```python
from build123d import *

# Parameters (mm, degrees)
F0_W     = 50.8
F0_H     = 1219.2
F1_DEPTH = 25.4


with BuildPart() as f1:
    # F0 (on Right) → F1 (new body)
    with BuildSketch(Plane.YZ):
        Polygon((350.804755, -361.721163), (350.804755, -336.321163), (-182.595245, -336.321163), (-233.395245, -336.321163), (-487.395245, -336.321163), (-538.195245, -336.321163), (-538.195245, -361.721163), align=None)
        with Locations((-207.995245, 273.278837)):
            Rectangle(F0_W, F0_H)
        Polygon((-233.395245, 882.878837), (-182.595245, 882.878837), (-182.595245, 908.278837), (-538.195245, 908.278837), (-538.195245, 882.878837), (-487.395245, 882.878837), align=None)
        with Locations((-512.795245, 273.278837)):
            Rectangle(F0_W, F0_H)
    extrude(amount=F1_DEPTH)


solid = f1.part
```
Work out the finished part from the listing and answer in its coordinate system (mm). A direction names the side the tool comes from. Give positions to 0.01 mm unless a question says otherwise; leave off trailing zeros. Loops run counter-clockwise (first coordinate to the right, second up) from the corner with the lowest first, then second, coordinate; pieces in that order, holes last. Notation, with made-up numbers: (34, 45.25) -> (56, 45.25) arc R6 cw to (56, 53.25) -> close; hole circle Ø3 at (1, 80.25). An arc over 180 degrees is marked (long way). Put each result on its own line as item: value. Start each with the question number.
Item 1: Which of the six approach directions +Z, -Z, +X, -X, +Y, -Y give full straight-line access (tool end or side, diameter ignored) to faces 5 (the face through (13, -358, 908.279)), 6 (the face through (13, 88, -336.321)), 7 (the face through (13, -362, 882.879))?
Item 2: The part is cut by section B-B (x = 7.75). Give the vertices of the cut face in (y, z).
Item 3: The mould has two halves that part along Y. Classify faces 1 (the face through (13, -182.595, 277)), 2 (the face through (13, -233.395, 265)), 3 (the face through (13, -359, -336.321)), 4 (the face through (13, -100, -361.721)): released by +Y, released by -Y, zero draft, split by the parting line, or undercut.
Item 4: The part is cut by section A-A (z = 518). Give the vertices of the cut face in (x, y).
Item 5: Each of these flat-tipped pins is pushed along its axis until it touches: P1, Ø10, axis at x = 5.5, y = 79, coming from the +Z side; P2, Ø7.5, axis at x = 13, z = 123.5, coming from the +Y side. Where does it stop, or does it pass through?
Item 6: Find the intervals of material crossed by L1, parallel to Y at x = 21, z = 135; L2, parallel to Z at x = 18, y = -329; L3, parallel to Z at x = 11.5, y = -72, in increasing order. Write a range as [from, to].
Item 7: The part is cut by section C-C (y = 273). Give the vertices of the cut face in (x, z).
Answers below:
1. face 5: +Z, +X, -X, +Y, -Y
1. face 6: +Z, +X, -X, +Y
1. face 7: +X, -X
2. outline: (-538.2, -361.72) -> (350.8, -361.72) -> (350.8, -336.32) -> (-182.6, -336.32) -> (-182.6, 908.28) -> (-538.2, 908.28) -> close; hole (-487.4, -336.32) -> (-233.4, -336.32) -> (-233.4, 882.88) -> (-487.4, 882.88) -> close
3. face 1: released by +Y
3. face 2: undercut
3. face 3: undercut
3. face 4: zero draft
4. outline: (0, -538.2) -> (25.4, -538.2) -> (25.4, -487.4) -> (0, -487.4) -> close; (0, -233.4) -> (25.4, -233.4) -> (25.4, -182.6) -> (0, -182.6) -> close
5. P1: z = -336.32
5. P2: y = -182.6
6. L1: [-538.2, -487.4], [-233.4, -182.6]
6. L2: [-361.72, -336.32], [882.88, 908.28]
6. L3: [-361.72, -336.32]
7. outline: (0, -361.72) -> (25.4, -361.72) -> (25.4, -336.32) -> (0, -336.32) -> close
